```python
from build123d import *

# Parameters (mm, degrees)
SKETCH1_W           = 14
SKETCH1_H           = 40
BOSS_EXTRUDE1_DEPTH = 3.175


with BuildPart() as part:
    # Sketch1 → Boss-Extrude1 (new body)
    with BuildSketch(Plane(origin=(0, 0, 0), x_dir=(1, 0, 0), z_dir=(0, 1, 0))):
        Polygon((-17.875, -38.1), (-14.7, -38.1), (-14.7, -53.51285), (14.7, -53.51285), (14.7, -38.1), (17.875, -38.1), (17.875, -12.7), (14.7, -12.7), (14.7, 12.7), (17.875, 12.7), (17.875, 38.1), (14.7, 38.1), (14.7, 53.51285), (-14.7, 53.51285), (-14.7, 38.1), (-17.875, 38.1), (-17.875, 12.7), (-14.7, 12.7), (-14.7, -12.7), (-17.875, -12.7), align=None)
        Rectangle(SKETCH1_W, SKETCH1_H, mode=Mode.SUBTRACT)
        Polygon((-21.05, -38.1), (-17.875, -38.1), (-17.875, -12.7), (-17.875, 12.7), (-17.875, 38.1), (-21.05, 38.1), align=None)
        Polygon((17.875, -12.7), (17.875, -38.1), (21.05, -38.1), (21.05, 38.1), (17.875, 38.1), (17.875, 12.7), align=None)
    extrude(amount=BOSS_EXTRUDE1_DEPTH)


solid = part.part
```
Can you work these out from the model? Positions are in its coordinate system, mm. A direction names the side the tool comes from. Give positions to 0.01 mm unless a question says otherwise; leave off trailing zeros. Loops run counter-clockwise (first coordinate to the right, second up) from the corner with the lowest first, then second, coordinate; pieces in that order, holes last. Notation, with made-up numbers: M 30,56 L 53,56 A34 cw 53,94 Z; hole C 64.25,-4 d4. An arc over 180 degrees is marked long. Use one line per item in the form item = value. Start each with the question number.
(1) Thinking about a two-plate mould opening in Z: for faces 1 (the flat face through (18, 2, 38.1)), 2 (the flat face through (0, 2, -53.513)), 3 (the flat face through (21.05, 2, 1)), 4 (the flat face through (0, 2, -20)), which applies, released by +Z, released by -Z, zero draft, split by the parting line, or undercut?
(2) I want a section at B-B, the plane z = -10. Write out the boundary of the cut face in (x, y) (3 decimals).
(3) Please list where these lines run through material, in increasing order: line 1 (X direction, y = 0.7, z = -4) (3 decimals); line 2 (Z direction, x = 16, y = 1.65); line 3 (Z direction, x = 5.5, y = 2.6).
(4) I want a section at C-C, the plane z = 18.5. Write out the boundary of the cut face in (x, y) (3 decimals), and give its area (3 significant figures).
(5) I want a section at A-A, the plane y = 2. Write out the boundary of the cut face in (x, z) (3 decimals), and give its area (3 significant figures).
(6) I want a section at D-D, the plane z = 46. Write out the boundary of the cut face in (x, y) (3 decimals).
(7) I'm going to push flat-ended pins straight in: P1, Ø1, axis at x = 16.5, y = 1.5, coming from the +Z side; P2, Ø1.6, axis at x = -16.5, y = 1.5, coming from the -Z side. Where does each tip first touch, or does it pass through?
(8) On a 3-axis mill with a long thin cutter (end or side, diameter ignored), from which of +Z, -Z, +X, -X, +Y, -Y can I reach the whole of each face in a straight line? I mean faces 5 (the flat face through (-14.7, 2, 46)), 6 (the flat face through (9, 0, -1)), 7 (the flat face through (-14.7, 2, -46)), 8 (the flat face through (16, 2, -12.7)), 9 (the flat face through (14.7, 2, -46)). Say none if no direction works.
Worked out:
q1.face_1 = released by +Z
q1.face_2 = released by -Z
q1.face_3 = zero draft
q1.face_4 = undercut
q2.outline = M -21.05,0 L -17.875,0 L -17.875,3.175 L -21.05,3.175 Z; M -14.7,0 L -7,0 L -7,3.175 L -14.7,3.175 Z; M 7,0 L 14.7,0 L 14.7,3.175 L 7,3.175 Z; M 17.875,0 L 21.05,0 L 21.05,3.175 L 17.875,3.175 Z
q3.line_1 = -21.05 to -17.875, -14.7 to -7, 7 to 14.7, 17.875 to 21.05
q3.line_2 = -38.1 to -12.7, 12.7 to 38.1
q3.line_3 = -53.51 to -20, 20 to 53.51
q4.outline = M -21.05,0 L -7,0 L -7,3.175 L -21.05,3.175 Z; M 7,0 L 21.05,0 L 21.05,3.175 L 7,3.175 Z
q4.area = 89.2 mm²
q5.outline = M -21.05,-38.1 L -14.7,-38.1 L -14.7,-53.513 L 14.7,-53.513 L 14.7,-38.1 L 21.05,-38.1 L 21.05,38.1 L 14.7,38.1 L 14.7,53.513 L -14.7,53.513 L -14.7,38.1 L -21.05,38.1 Z; hole M -17.875,-12.7 L -14.7,-12.7 L -14.7,12.7 L -17.875,12.7 Z; hole M -7,-20 L 7,-20 L 7,20 L -7,20 Z; hole M 14.7,-12.7 L 17.875,-12.7 L 17.875,12.7 L 14.7,12.7 Z
q5.area = 3,390 mm²
q6.outline = M -14.7,0 L 14.7,0 L 14.7,3.175 L -14.7,3.175 Z
q7.P1 = 38.1
q7.P2 = -38.1
q8.face_5 = +Z, -X, +Y, -Y
q8.face_6 = +Z, -Z, +X, -X, -Y
q8.face_7 = -Z, -X, +Y, -Y
q8.face_8 = +Y, -Y
q8.face_9 = -Z, +X, +Y, -Y
